from build123d import *

# Parameters (mm, degrees)
F0_W     = 23.84
F0_H     = 1.58
F1_DEPTH = 7
F2_R     = 1.5
F2_W     = 5.92
F2_H     = 7
F3_DEPTH = 25
F4_R     = 1.5
F4_W     = 5.92
F4_H     = 7
F5_DEPTH = 25


with BuildPart() as f1:
    # F0 (on Top) → F1 (new body)
    with BuildSketch(Plane.XY):
        Polygon((0, 25.42), (0, 0), (1.58, 0), (1.58, 1.58), (1.58, 25.42), align=None)
        with Locations((13.5, 0.79)):
            Rectangle(F0_W, F0_H)
    extrude(amount=F1_DEPTH)

    # F2 (on face) → F3 (cut)
    with BuildSketch(Plane(origin=(0, 0, 0), x_dir=(0, -1, 0), z_dir=(-1, 0, 0))):
        with Locations((-15, 3.5)):
            Circle(F2_R)
        with Locations((-22.46, 3.5)):
            Rectangle(F2_W, F2_H)
    extrude(amount=-F3_DEPTH, mode=Mode.SUBTRACT)

    # F4 (on face) → F5 (cut)
    with BuildSketch(Plane.XZ):
        with Locations((15, 3.5)):
            Circle(F4_R)
        with Locations((22.46, 3.5)):
            Rectangle(F4_W, F4_H)
    extrude(amount=-F5_DEPTH, mode=Mode.SUBTRACT)


solid = f1.part
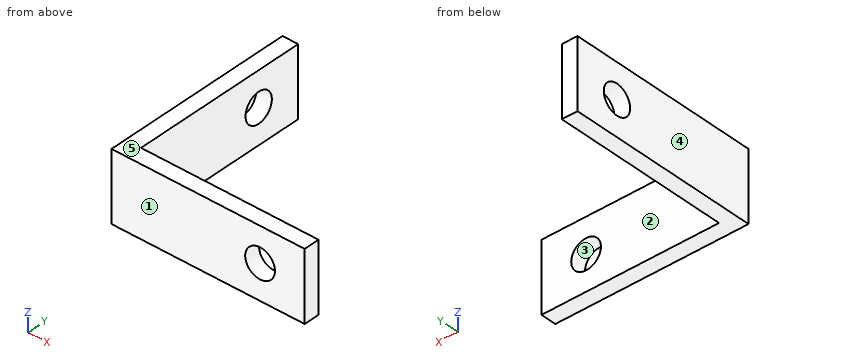
Geometry: final body of the model. Coordinates: model frame, mm. Face numbers are marked on the shaded views. A direction names the side the tool comes from. Coordinates: 2 decimals unless noted, no trailing zeros. Order: outer loops, then holes, each group sorted by start corner. A loop starts at its lowest first (then second) coordinate and runs counter-clockwise, first axis right, second up.
1) Section A-A (z = 3.5). Return loops of the section in (x, y), then the cut area to 3 significant figures.
Result sheet:
outline: (0, 0) - (13.5, 0) - (13.5, 1.58) - (1.58, 1.58) - (1.58, 13.5) - (0, 13.5) - close; (0, 16.5) - (1.58, 16.5) - (1.58, 19.5) - (0, 19.5) - close; (16.5, 0) - (19.5, 0) - (19.5, 1.58) - (16.5, 1.58) - close
area: 49.6 mm2
2) Section B-B (x = 15). Return loops of the section in (y, z).
Result sheet:
outline: (0, 0) - (1.58, 0) - (1.58, 2) - (0, 2) - close; (0, 5) - (1.58, 5) - (1.58, 7) - (0, 7) - close
3) Section D-D (z = 1.5). Return loops of the section in (x, y).
Result sheet:
outline: (0, 0) - (19.5, 0) - (19.5, 1.58) - (1.58, 1.58) - (1.58, 19.5) - (0, 19.5) - close
4) Draft query along Z for the marked faces 3, 4 and 5. Return one class per face: released by +Z, released by -Z, zero draft, split by the parting line, or undercut.
Result sheet:
face 3: undercut
face 4: zero draft
face 5: released by +Z
5) Set-up query: the marked faces 1 and 2. Return all of +Z, -Z, +X, -X, +Y, -Y with unobstructed straight access to the full face (end or side cutting, diameter ignored); none if empty.
Result sheet:
face 1: +Z, -Z, +X, -X, -Y
face 2: +Z, -Z, +X, +Y
6) Ray query, probe 1 along Z at (x, y) = (15, 0.7); probe 2 along Y at (x, z) = (3.75, 6.25). Return the intervals inside material, ascending.
Result sheet:
probe 1: z = 0 to 2, 5 to 7
probe 2: y = 0 to 1.58
7) First-contact query: P1, Ø3.5, axis at y = 10, z = 2, coming from the +X side. Flat tip, straight axial feed; report the tip coordinate or a pass-through.
Result sheet:
P1: stops at x = 1.58
